Can you work these out from the model? Positions are in its coordinate system, mm. Give positions to 0.01 mm unless a question says otherwise; leave off trailing zeros. Write each loop counter-clockwise with the first axis right and the second up, starting at its lowest first coordinate (ties: lowest second). Pieces come first, ordered by that corner, then holes. Notation, with made-up numbers: (84, 57.25) - (135, 57.25) arc R19 ccw to (135, 86.25) - close; hole circle Ø4 at (-18, -37.75). An arc over 180 degrees is marked (long way). Use a Markdown table: item, result. Add a question column.
Autodesk Inventor part; units mm, degrees
ref_plane "YZ Plane" through (0, 0, 0) normal (1, 0, 0) x (0, 1, 0)
ref_plane "XZ Plane" through (0, 0, 0) normal (0, 1, 0) x (-1, 0, 0)
ref_plane "XY Plane" through (0, 0, 0) normal (0, 0, 1) x (1, 0, 0)
sketch "Sketch1" plane through (0, 0, 0) normal (0, 1, 0) x (-1, 0, 0)
  line L0 (-33, 20) -> (0, 20)
  line L1 (0, 20) -> (0, 0) construction
  line L2 (0, 0) -> (-33, 0) construction
  line L3 (-33, 0) -> (-33, 20)
  line L4 (-37.8717, 14) -> (4.6091, 14) construction
  circle A0 centre (-12, 14) radius 2
  circle A1 centre (-27, 14) radius 2
  line L5 (33, 20) -> (0, 20)
  line L6 (33, 0) -> (33, 20)
  line L7 (37.8717, 14) -> (-4.6091, 14) construction
  circle A2 centre (12, 14) radius 2
  circle A3 centre (27, 14) radius 2
  line L8 (-33, -20) -> (0, -20)
  line L9 (0, -20) -> (0, 0) construction
  line L10 (-33, 0) -> (-33, -20)
  line L11 (-37.8717, -14) -> (4.6091, -14) construction
  circle A4 centre (-12, -14) radius 2
  circle A5 centre (-27, -14) radius 2
  line L12 (33, -20) -> (0, -20)
  line L13 (37.8717, -14) -> (-4.6091, -14) construction
  circle A6 centre (12, -14) radius 2
  circle A7 centre (27, -14) radius 2
  line L14 (33, 0) -> (33, -20)
  dimension "d0" = 33
  dimension "d1" = 20
  dimension "d2" = 6
  dimension "Bracket_Hole_Diameter" = 4
  dimension "d4" = 6
  dimension "d5" = 21
extrude "Plate1" add sketch "Sketch1" along normal blind 1
equation "\"BendRadius\" = Thickness"
equation "\"BendReliefWidth\" = Thickness"
equation "\"BendReliefDepth\" = 0.5 * Thickness"
equation "\"CornerReliefSize\" = 4 * Thickness"
equation "\"MinimumRemnant\" = 2 * Thickness"
equation "\"TransitionRadius\" = BendRadius"
equation "\"JacobiRadiusSize\" = BendRadius"
equation "\"GapSize\" = Thickness"
equation "\"d6\" = BendRadius"
equation "\"Bracket_Holes_LateralDistance\" = 28"
equation "\"Bracket_Holes_Distance\" = 15"
equation "\"Bracket_Holes_UnfoldedDistance\" = 24"
properties part number "BracketUnfolded" material "Steel, Galvanized"
Q1. I'm going to push a flat-ended pin straight in: P1, Ø5, axis at x = -12, z = -14, coming from the +Y side. Where does the tip first touch, or does it pass through?
Q2. Suppose I cut it at C-C (y = 0.45). Give the number of separate pieces and of enclosed holes in the cut face, and give its area (3 significant figures).
Q3. If we mould it in two halves opening along X, with no side actions, what happens to faces 1 (the cylindrical face through (-10.526, 0.493, -15.352)), 2 (the flat face through (0, 0, 0))? For each: released by +X, released by -X, zero draft, split by the parting line, or undercut.
Q4. Suppose I cut it at B-B (x = 12). Please give me the cut outline in (y, z), and give its area (3 significant figures).
Q5. If I drill on probe 1 along Z at (x, y) = (27, 0.65); probe 2 along X at (y, z) = (0.7, 13.5); probe 3 along Z at (x, y) = (-13.5, 0.1), over which ranges is the centre line in solid material (lowest first)? Write a range as [from, to].
Q6. Suppose I cut it at A-A (z = -14). Please give me the cut outline in (x, y), and give its area (3 significant figures).
Derived:
| question | item | result |
|---|---|---|
| 1 | P1 | y = 1 |
| 2 | separate pieces | 1 |
| 2 | enclosed holes | 8 |
| 2 | area | 2,540 mm² |
| 3 | face 1 | undercut |
| 3 | face 2 | zero draft |
| 4 | outline | (0, -20) - (1, -20) - (1, -16) - (0, -16) - close; (0, -12) - (1, -12) - (1, 12) - (0, 12) - close; (0, 16) - (1, 16) - (1, 20) - (0, 20) - close |
| 4 | area | 32.0 mm² |
| 5 | probe 1 | [-20, -16], [-12, 12], [16, 20] |
| 5 | probe 2 | [-33, -28.94], [-25.06, -13.94], [-10.06, 10.06], [13.94, 25.06], [28.94, 33] |
| 5 | probe 3 | [-20, -15.32], [-12.68, 12.68], [15.32, 20] |
| 6 | outline | (-33, 0) - (-29, 0) - (-29, 1) - (-33, 1) - close; (-25, 0) - (-14, 0) - (-14, 1) - (-25, 1) - close; (-10, 0) - (10, 0) - (10, 1) - (-10, 1) - close; (14, 0) - (25, 0) - (25, 1) - (14, 1) - close; (29, 0) - (33, 0) - (33, 1) - (29, 1) - close |
| 6 | area | 50.0 mm² |
